Check sheet for the drawn part. Datum: minimum x, y, z corner. Units: mm. A direction names the side the tool comes from. Give positions to 0.01 mm unless a question says otherwise; leave off trailing zeros. Loops run counter-clockwise (first coordinate to the right, second up) from the corner with the lowest first, then second, coordinate; pieces in that order, holes last. Notation, with made-up numbers: (-25, 78.25) - (-15, 78.25) arc R10 ccw to (-15, 94.25) - close; hole circle Ø11 at (6, 58). An arc over 180 degrees is marked (long way). Answer in a Markdown table with one row per item.
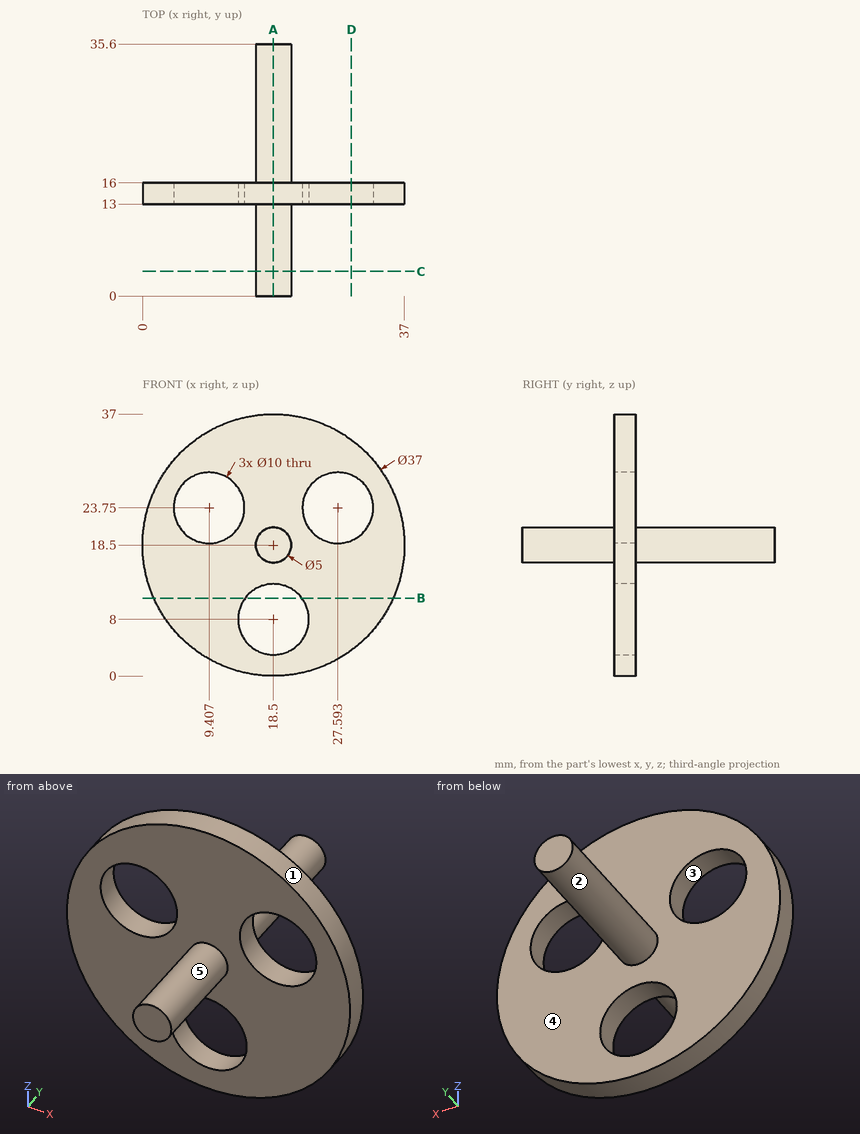
Q1. Go/stop test with flat-tipped pins: P1, Ø2, axis at y = 11.5, z = 23, coming from the -X side; P2, Ø2, axis at x = 22, z = 23, coming from the +Y side; P3, Ø12, axis at x = 4.5, y = 16, coming from the +Z side. Record where each tip stops, or that it passes through.
Completed:
| item | result |
|---|---|
| P1 | through |
| P2 | y = 16 |
| P3 | z = 35.18 |
Q2. Thickness scan on line 1 (X direction, y = 13.6, z = 23.75); line 2 (Z direction, x = 18, y = 14) (1 decimal); line 3 (Y direction, x = 13, z = 3). Record the ranges inside material, lowest first.
Completed:
| item | result |
|---|---|
| line 1 | 0.76 to 4.41, 14.41 to 22.59, 32.59 to 36.24 |
| line 2 | 0 to 3, 13 to 37 |
| line 3 | 13 to 16 |
Q3. Sectioned sample at B-B (z = 11). Record the cut outline in (x, y).
Completed:
| item | result |
|---|---|
| outline | (1.59, 13) - (14.5, 13) - (14.5, 16) - (1.59, 16) - close; (22.5, 13) - (35.41, 13) - (35.41, 16) - (22.5, 16) - close |
Q4. Sectioned sample at A-A (x = 18.5). Record the cut outline in (y, z), and give its area (3 significant figures).
Completed:
| item | result |
|---|---|
| outline | (0, 16) - (13, 16) - (13, 13) - (16, 13) - (16, 16) - (35.6, 16) - (35.6, 21) - (16, 21) - (16, 37) - (13, 37) - (13, 21) - (0, 21) - close; (13, 0) - (16, 0) - (16, 3) - (13, 3) - close |
| area | 244 mm^2 |
Q5. Sectioned sample at C-C (y = 3.5). Record the cut outline in (x, z).
Completed:
| item | result |
|---|---|
| outline | circle Ø5 at (18.5, 18.5) |
Q6. Tool access check on the marked faces 1 and 2. Record the directions out of +Z, -Z, +X, -X, +Y, -Y that give a thin tool (end or side, any length) a straight path to the whole face; none if there is none.
Completed:
| item | result |
|---|---|
| face 1 | +Y, -Y |
| face 2 | +Y |
Q7. Sectioned sample at D-D (x = 29.5). Record the cut outline in (y, z) (1 decimal).
Completed:
| item | result |
|---|---|
| outline | (13, 3.6) - (16, 3.6) - (16, 19.1) - (13, 19.1) - close; (13, 28.4) - (16, 28.4) - (16, 33.4) - (13, 33.4) - close |
Q8. Draft check along X on the marked faces 3, 4 and 5. Enter one of: +X half, -X half, draft (parallel to the pull), parting line (faces both ways), or undercut.
Completed:
| item | result |
|---|---|
| face 3 | undercut |
| face 4 | draft |
| face 5 | parting line |
